Autodesk Inventor part; units mm, degrees
ref_plane "YZ Plane" through (0, 0, 0) normal (1, 0, 0) x (0, 1, 0)
ref_plane "XZ Plane" through (0, 0, 0) normal (0, 1, 0) x (-1, 0, 0)
ref_plane "XY Plane" through (0, 0, 0) normal (0, 0, 1) x (1, 0, 0)
sketch "Sketch1" plane through (0, 0, 0) normal (0, 0, 1) x (1, 0, 0)
  line L0 (15, 0) -> (95, 0)
  line L1 (110, 15) -> (110, 15)
  line L2 (95, 30) -> (15, 30)
  line L3 (0, 15) -> (0, 15)
  circle A0 centre (10, 15) radius 5
  circle A1 centre (100, 15) radius 5
  arc A2 (110, 15) -> (95, 30) centre (95, 15) ccw
  arc A3 (95, 0) -> (110, 15) centre (95, 15) ccw
  arc A4 (0, 15) -> (15, 0) centre (15, 15) ccw
  arc A5 (15, 30) -> (0, 15) centre (15, 15) ccw
  point P0 (0, 0)
  point P1 (110, 0)
  point P2 (110, 30)
  point P3 (0, 15)
  dimension "d1" = 30
  dimension "d14" = 10
  dimension "d15" = 10
  dimension "d16" = 10
  dimension "d17" = 90
  dimension "d18" = 15
  dimension "d21" = 15
extrude "Extrusion1" add sketch "Sketch1" along normal blind 3
sketch "Sketch2" plane through (0, 0, 3) normal (0, 0, 1) x (1, 0, 0)
  arc A0 (95, 0) -> (95, 30) centre (95, 15) ccw
  line L0 (95, 30) -> (15, 30)
  arc A1 (15, 30) -> (15, 0) centre (15, 15) ccw
  line L1 (15, 0) -> (95, 0)
  circle A2 centre (100, 15) radius 5
  circle A3 centre (10, 15) radius 5
  circle A4 centre (100, 15) radius 5
  line L2 (15, 0) -> (95, 0)
  line L3 (95, 30) -> (15, 30)
  circle A5 centre (112, 15) radius 30
  point P0 (0, 0)
  point P1 (86.0192, 0)
  point P2 (86.0192, 30)
  dimension "d32" = 60
  dimension "d33" = 12
extrude "Extrusion2" add sketch "Sketch2" along normal blind 6 contours L1 A1 L0 A5
sketch "Sketch3" plane through (0, 0, 0) normal (0, 0, -1) x (-1, 0, 0)
  arc A0 (-95, 30) -> (-95, 0) centre (-95, 15) ccw
  line L0 (-15, 0) -> (-95, 0)
  arc A1 (-15, 0) -> (-15, 30) centre (-15, 15) ccw
  line L1 (-95, 30) -> (-15, 30)
  circle A2 centre (-100, 15) radius 5
  circle A3 centre (-10, 15) radius 5
  circle A4 centre (-50.5, 15) radius 5
  circle A5 centre (-70, 15) radius 5
  circle A6 centre (-10, 15) radius 5
  line L2 (-50.5, 20) -> (-70, 20)
  line L3 (-70, 10) -> (-50.5, 10)
  point P0 (0, 0)
  dimension "d26" = 40.5
  dimension "d27" = 30
  dimension "d28" = 10
extrude "Extrusion3" cut sketch "Sketch3" against normal up to surface (9 mm away) contours A4 | A4 L3 A5 L2 | A5
sketch "Sketch4" plane through (0, 0, 9) normal (0, 0, 1) x (1, 0, 0)
  line L0 (70, 10) -> (50.5, 10)
  arc A0 (50.5, 20) -> (50.5, 10) centre (50.5, 15) ccw
  line L1 (50.5, 20) -> (70, 20)
  arc A1 (70, 10) -> (70, 20) centre (70, 15) ccw
  line L2 (15, 0) -> (86.0192, 0)
  arc A2 (86.0192, 30) -> (86.0192, 0) centre (112, 15) ccw
  line L3 (86.0192, 30) -> (15, 30)
  arc A3 (15, 30) -> (15, 0) centre (15, 15) ccw
  circle A4 centre (10, 15) radius 5
  circle A5 centre (70, 15) radius 15
  line L4 (15, 0) -> (95, 0)
  circle A6 centre (70, 15) radius 30
  point P0 (0, 0)
  point P1 (44.0192, 0)
  point P2 (44.0192, 30)
  dimension "d34" = 60
  dimension "d35" = 60
extrude "Extrusion4" add sketch "Sketch4" along normal blind 6 contours L2 A3 L3 A6
sketch "Sketch5" plane through (0, 0, 0) normal (0, 0, -1) x (-1, 0, 0)
  circle A0 centre (-30.25, 15) radius 2.5
  arc A1 (-50.5, 10) -> (-50.5, 20) centre (-50.5, 15) ccw
  circle A2 centre (-10, 15) radius 5
  point P0 (0, 0)
  dimension "d38" = 5
  dimension "d39" = 40.5
  dimension "d40" = 20.25
extrude "Extrusion5" cut sketch "Sketch5" against normal blind 0.1 contours A0
equation "\"d14\" = d6"
equation "\"d15\" = d14"
equation "\"d16\" = d15"
equation "\"d18\" = 0.5 * d1"
equation "\"d21\" = 0.5 * d1"
equation "\"d19\" = d11"
equation "\"d32\" = 2 * d0"
equation "\"d33\" = 0.4 * d0"
equation "\"d22\" = 2 * d11"
equation "\"d26\" = 1.35 * d0"
equation "\"d27\" = d0"
equation "\"d34\" = 2 * d0"
equation "\"d35\" = 2 * d0"
equation "\"d36\" = 2 * d11"
equation "\"d40\" = 0.5 * d39"
properties part number "GripP4"
Here's how the part is built. I have some questions about the finished solid (model axes, mm). A direction names the side the tool comes from. Coordinates: 2 decimals unless noted, no trailing zeros. Loops run counter-clockwise (first coordinate to the right, second up) from the corner with the lowest first, then second, coordinate; pieces in that order, holes last. Notation, with made-up numbers: (-13.5, -39) -> (16.5, -39) arc R3 cw to (16.5, -34) -> close; hole circle Ø6 at (-26, 50). An arc over 180 degrees is marked (long way). Use one line per item in the form item = value. Start each with the question number.
(1) If we section it at B-B (x = 10): Please give me the cut outline in (y, z), then the cut area to 3 significant figures.
(2) If we section it at D-D (x = 79): Please give me the cut outline in (y, z).
(3) Please list where these lines run through material, in increasing order: line 1 along Y through (x, z) = (67, 8.75); line 2 along Y through (x, z) = (30.25, 0.05); line 3 along X through (y, z) = (19, 5).
(4) If we section it at A-A (z = 13): Please give me the cut outline in (x, y).
(5) We'd pull the mould along Y, two halves only. Please class faces 1 (the face through (0, 15, 7)), 2 (the face through (54, 22, 0)), 3 (the face through (75, 15, 4)), 4 (the face through (60, 10, 4)): pulls with the +Y half, pulls with the -Y half, needs draft (parallel to the pull), parting line crosses it, or undercut.
(6) If we section it at C-C (y = 6): Please give me the cut outline in (x, z).
(7) Will these pins go through, and if not, where does the flat tip stop? pin 1 (8.5 mm diameter, centred on x = 97, y = 7.5, fed in from +Z); pin 2 (9 mm diameter, centred on x = 69.5, y = 21.5, fed in from +Z).
(8) On a 3-axis mill with a long thin cutter (end or side, diameter ignored), from which of +Z, -Z, +X, -X, +Y, -Y can I reach the whole of each face in a straight line? I mean faces 5 (the face through (45.5, 14.9, 4.4)), 6 (the face through (63, 22, 9)), 7 (the face through (30, 15, 0.1)). Say none if no direction works.
Verdict:
q1.outline = (0.86, 0) -> (10, 0) -> (10, 15) -> (0.86, 15) -> close; (20, 0) -> (29.14, 0) -> (29.14, 15) -> (20, 15) -> close
q1.area = 274 mm²
q2.outline = (0, 0) -> (30, 0) -> (30, 9) -> (0, 9) -> close
q3.line_1 = 0 to 10, 20 to 30
q3.line_2 = 0 to 12.5, 17.5 to 30
q3.line_3 = 0.54 to 7, 13 to 47.5, 73 to 82.27
q4.outline = (15, 0) -> (44.02, 0) arc R30 cw to (44.02, 30) -> (15, 30) arc R15 ccw to start; hole circle Ø10 at (10, 15)
q5.face_1 = parting line crosses it
q5.face_2 = needs draft
q5.face_3 = undercut
q5.face_4 = undercut
q6.outline = (3, 0) -> (107, 0) -> (107, 3) -> (83.38, 3) -> (83.38, 9) -> (41.38, 9) -> (41.38, 15) -> (3, 15) -> close
q7.pin_1 = 3
q7.pin_2 = 9
q8.face_5 = +Z, -Z
q8.face_6 = +Z, +X
q8.face_7 = -Z
